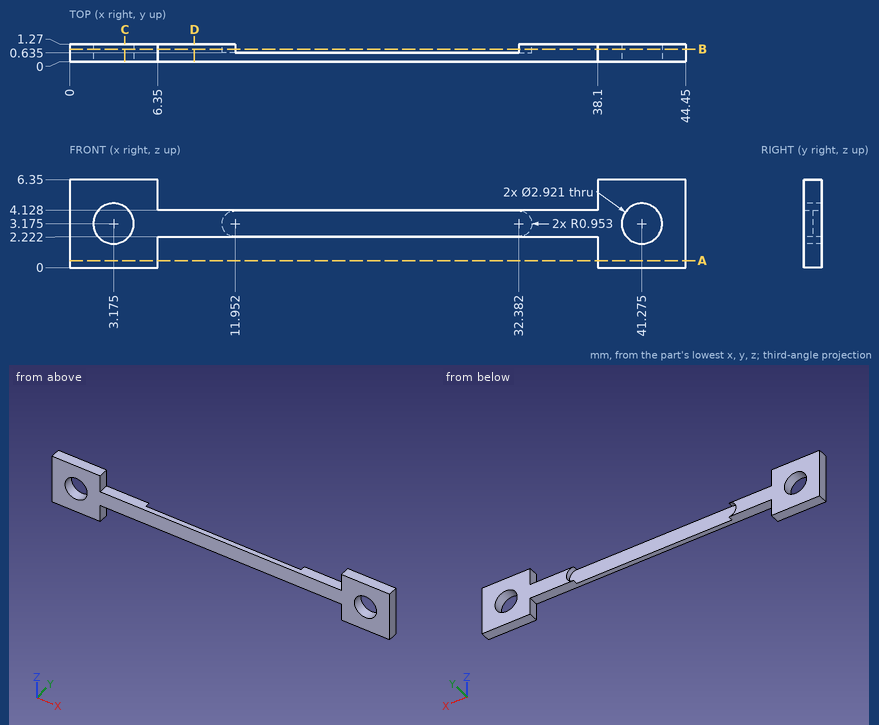
Answer from the drawing. Dimensions are ordinates in mm from the lowest x, y and z of the part. Round coordinates to 2 decimals unless told otherwise and drop trailing zeros. Loops run counter-clockwise (first coordinate to the right, second up) from the corner with the lowest first, then second, coordinate; pieces in that order, holes last.
1) A cutting plane is placed at D-D on x = 9. Determine the outline of the cut face in (y, z).
Outcome:
outline: (0, 2.22) - (1.27, 2.22) - (1.27, 4.13) - (0, 4.13) - close
2) A cutting plane is placed at A-A on z = 0.5. Determine the outline of the cut face in (x, y).
Outcome:
outline: (0, 0) - (6.35, 0) - (6.35, 1.27) - (0, 1.27) - close; (38.1, 0) - (44.45, 0) - (44.45, 1.27) - (38.1, 1.27) - close
3) A cutting plane is placed at B-B on y = 0.9. Give the number of separate pieces and of enclosed holes in the cut face.
Outcome:
separate pieces: 2
enclosed holes: 2
4) Given P1, Ø2, axis at x = 30, z = 5.5, coming from the -Y side; P2, Ø1.5, axis at x = 23, z = 3, coming from the +Y side (1 decimal), each flat-ended and moving along its own axis, determine where each tip first touches the part or whether it passes through.
Outcome:
P1: passes through
P2: stops at y = 0.6
5) Consider line 1 (X direction, y = 0.45, z = 3.25); line 2 (X direction, y = 0.4, z = 6); line 3 (X direction, y = 0.45, z = 2.5). Determine where each line is inside the solid, lowest interval first.
Outcome:
line 1: x = 0 to 1.72, 4.63 to 39.82, 42.73 to 44.45
line 2: x = 0 to 6.35, 38.1 to 44.45
line 3: x = 0 to 1.88, 4.47 to 39.98, 42.57 to 44.45
6) A cutting plane is placed at C-C on x = 4. Determine the outline of the cut face in (y, z).
Outcome:
outline: (0, 0) - (1.27, 0) - (1.27, 1.97) - (0, 1.97) - close; (0, 4.38) - (1.27, 4.38) - (1.27, 6.35) - (0, 6.35) - close
